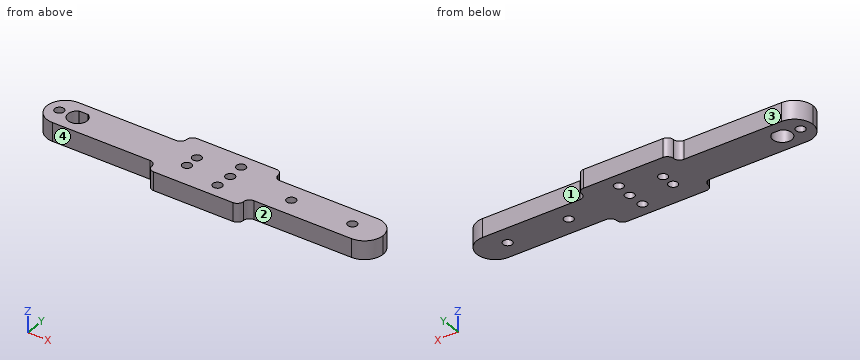
Autodesk Inventor part; units mm, degrees
ref_plane "YZ Plane" through (0, 0, 0) normal (1, 0, 0) x (0, 1, 0)
ref_plane "XZ Plane" through (0, 0, 0) normal (0, 1, 0) x (-1, 0, 0)
ref_plane "XY Plane" through (0, 0, 0) normal (0, 0, 1) x (1, 0, 0)
sketch "Sketch1" plane through (0, 0, 0) normal (0, 0, 1) x (1, 0, 0)
  line L0 (0, 0) -> (90, 0) construction
  line L1 (0, -10) -> (90, -10)
  line L2 (90, 10) -> (0, 10)
  arc A0 (0, 10) -> (0, -10) centre (0, 0) ccw
  arc A1 (90, -10) -> (90, 10) centre (90, 0) ccw
  line L3 (0, 0) -> (90, 0) construction
  circle A2 centre (0, 0) radius 3.1
  circle A3 centre (-6, 0) radius 1.5
  circle A4 centre (0, 0) radius 37.5 construction
  circle A5 centre (0, 0) radius 50 construction
  circle A6 centre (37.4301, 2.2893) radius 1.5
  circle A7 centre (37.4301, -2.2893) radius 1.5
  circle A8 centre (50, 0) radius 1.5
  circle A9 centre (49.7028, 5.4433) radius 1.5
  circle A10 centre (49.7028, -5.4433) radius 1.5
  line L4 (37.4301, 2.2893) -> (0, 0) construction
  line L5 (0, 0) -> (49.7028, 5.4433) construction
  line L6 (37.4301, -2.2893) -> (0, 0) construction
  line L7 (49.7028, -5.4433) -> (0, 0) construction
  circle A11 centre (90, 0) radius 1.5
  line L8 (-10, 10) -> (10, 10)
  line L9 (10, 10) -> (10, -10)
  line L10 (10, -10) -> (-10, -10)
  line L11 (-10, -10) -> (-10, 10)
  line L12 (-10, 10) -> (10, -10) construction
  line L13 (10, 10) -> (-10, -10) construction
  line L14 (80, 10) -> (100, 10)
  line L15 (100, 10) -> (100, -10)
  line L16 (100, -10) -> (80, -10)
  line L17 (80, -10) -> (80, 10)
  line L18 (80, 10) -> (100, -10) construction
  line L19 (100, 10) -> (80, -10) construction
  line L20 (30, 10) -> (60, 10)
  line L21 (60, 10) -> (60, -10)
  line L22 (60, -10) -> (30, -10)
  line L23 (30, -10) -> (30, 10)
  line L24 (30, 10) -> (60, -10) construction
  line L25 (60, 10) -> (30, -10) construction
  line L26 (-10, 6) -> (100, 6)
  line L27 (100, 6) -> (100, -6)
  line L28 (100, -6) -> (-10, -6)
  line L29 (-10, -6) -> (-10, 6)
  line L30 (-10, 6) -> (100, -6) construction
  line L31 (100, 6) -> (-10, -6) construction
  line L32 (-1.478, 2.725) -> (1.478, 2.725)
  circle A12 centre (70, 0) radius 1.5
  point P0 (45, 0)
  point P1 (30, 6)
  point P2 (30, -6)
  point P3 (60, -6)
  point P4 (60, 6)
  dimension "d0" = 90
  dimension "d1" = 0
  dimension "d2" = 20
  dimension "d4" = 6.2
  dimension "d5" = 3
  dimension "d6" = 6
  dimension "d7" = 0
  dimension "d8" = 75
  dimension "d9" = 100
  dimension "d10" = 3
  dimension "d11" = 3
  dimension "d12" = 3
  dimension "d13" = 3
  dimension "d14" = 3
  dimension "d15" = 3.5
  dimension "d16" = 3.5
  dimension "d17" = 6.25
  dimension "d18" = 6.25
  dimension "d19" = 3
  dimension "d22" = 20
  dimension "d23" = 20
  dimension "d24" = 20
  dimension "d25" = 20
  dimension "d26" = 30
  dimension "d27" = 20
  dimension "d28" = 12
  dimension "d31" = 2.725
  dimension "d32" = 3
  dimension "d33" = 20
  dimension "d34" = 0
extrude "Extrusion1" add sketch "Sketch1" along normal blind 6 contours L28 L11 A0 | A0 L26 L9 L28 | L23 L28 A10 L21 L1 | L9 L26 L23 L28 | L11 L26 A0 | L23 L26 A9 L21 L28 A10 | L21 L26 L17 L28 | L23 L2 L21 L26 A9 | L17 L26 A1 L28 | A1 L15 L28 | A1 L26 L15 | L32 A2 picked at (0.2541, 2.8183)
fillet "Fillet1" radius 2 8 edges at (30, 6, 3) (30, 10, 3) (60, 10, 3) (60, 6, 3) (60, -6, 3) (60, -10, 3) (30, -10, 3) (30, -6, 3)
fillet "Fillet1" radius 6 4 edges at (-10, -6, 3) (-10, 6, 3) (100, -6, 3) (100, 6, 3)
sketch "Sketch2" plane through (0, 0, 6) normal (0, 0, 1) x (1, 0, 0)
  arc A0 (94, -6) -> (94, 6) centre (94, 0) ccw
  line L0 (94, 6) -> (62, 6)
  arc A1 (60, 8) -> (62, 6) centre (62, 8) ccw
  arc A2 (60, 8) -> (58, 10) centre (58, 8) ccw
  line L1 (58, 10) -> (32, 10)
  arc A3 (32, 10) -> (30, 8) centre (32, 8) ccw
  arc A4 (28, 6) -> (30, 8) centre (28, 8) ccw
  line L2 (28, 6) -> (-4, 6)
  arc A5 (-4, 6) -> (-4, -6) centre (-4, 0) ccw
  line L3 (-4, -6) -> (28, -6)
  arc A6 (30, -8) -> (28, -6) centre (28, -8) ccw
  arc A7 (30, -8) -> (32, -10) centre (32, -8) ccw
  line L4 (32, -10) -> (58, -10)
  arc A8 (58, -10) -> (60, -8) centre (58, -8) ccw
  arc A9 (62, -6) -> (60, -8) centre (62, -8) ccw
  line L5 (62, -6) -> (94, -6)
  circle A10 centre (90, 0) radius 1.5
  circle A11 centre (70, 0) radius 1.5
  circle A12 centre (49.7028, 5.4433) radius 1.5
  circle A13 centre (50, 0) radius 1.5
  circle A14 centre (37.4301, -2.2893) radius 1.5
  circle A15 centre (37.4301, 2.2893) radius 1.5
  circle A16 centre (-6, 0) radius 1.5
  circle A17 centre (49.7028, -5.4433) radius 1.5
  line L6 (-1.478, 2.725) -> (1.478, 2.725)
  arc A18 (-1.478, 2.725) -> (1.478, 2.725) centre (0, 0) ccw
properties part number "Arm1_3D"
Work out the finished part from the listing and answer in its coordinate system (mm). Face numbers are marked on the shaded views. A direction names the side the tool comes from. Round coordinates to 2 decimals unless told otherwise and drop trailing zeros. Loops run counter-clockwise (first coordinate to the right, second up) from the corner with the lowest first, then second, coordinate; pieces in that order, holes last.
(1) Each of these flat-tipped pins is pushed along its axis until it touches: P1, Ø3.5, axis at x = 0, z = 2.5, coming from the -Y side; P2, Ø3, axis at x = 8, z = 4, coming from the +Y side; P3, Ø3.5, axis at x = 50, y = 0, coming from the -Z side; P4, Ø2, axis at y = -5.5, z = 3.5, coming from the -X side. Where does it stop, or does it pass through?
Computed values:
P1: stops at y = -6
P2: stops at y = 6
P3: stops at z = 0
P4: stops at x = -7.97
(2) The part is cut by section C-C, the plane x = 50. Give the vertices of the cut face in (y, z).
Computed values:
outline: (-10, 0) - (-6.91, 0) - (-6.91, 6) - (-10, 6) - close; (-3.97, 0) - (-1.5, 0) - (-1.5, 6) - (-3.97, 6) - close; (1.5, 0) - (3.97, 0) - (3.97, 6) - (1.5, 6) - close; (6.91, 0) - (10, 0) - (10, 6) - (6.91, 6) - close
(3) Find the intervals of material crossed by L1, parallel to X at y = -0.25, z = 4.3; L2, parallel to X at y = -5.25, z = 3.6; L3, parallel to Y at x = 84.5, z = 0.65, in increasing order.
Computed values:
L1: x = -9.99 to -7.48, -4.52 to -3.09, 3.09 to 48.52, 51.48 to 68.52, 71.48 to 88.52, 91.48 to 99.99
L2: x = -6.91 to 48.22, 51.19 to 96.91
L3: y = -6 to 6
(4) The part is cut by section B-B, the plane z = 2.1. Give the number of separate pieces and of enclosed holes in the cut face, and give its area (3 significant figures).
Computed values:
separate pieces: 1
enclosed holes: 9
area: 1,440 mm2
(5) The part is cut by section D-D, the plane x = 90.5. Give the vertices of the cut face in (y, z), and give its area (3 significant figures).
Computed values:
outline: (-6, 0) - (-1.41, 0) - (-1.41, 6) - (-6, 6) - close; (1.41, 0) - (6, 0) - (6, 6) - (1.41, 6) - close
area: 55.0 mm2
(6) The part is cut by section A-A, the plane x = 70. Give the vertices of the cut face in (y, z).
Computed values:
outline: (-6, 0) - (-1.5, 0) - (-1.5, 6) - (-6, 6) - close; (1.5, 0) - (6, 0) - (6, 6) - (1.5, 6) - close
(7) For the marked faces 1, 2, 3 and 4, determine the directions among +Z, -Z, +X, -X, +Y, -Y from which every point of the face is accessible in a straight line to the end or side of a thin tool.
Computed values:
face 1: +Z, -Z, +X, +Y
face 2: +Z, -Z, +X, -Y
face 3: +Z, -Z, -X, +Y
face 4: +Z, -Z, -X, -Y
